from build123d import *

# Parameters (mm, degrees)
BOSS_EXTRU_1_OUTLINE_W   = 46
BOSS_EXTRU_1_OUTLINE_H   = 46
BOSS_EXTRU_1_OUTLINE_W_2 = 5
BOSS_EXTRU_1_OUTLINE_H_2 = 5
BOSS_EXTRU_1_OUTLINE_R   = 5
BOSS_EXTRU_1_DEPTH       = 5
CONG_1_R                 = 3


# Read off the part's stored shape, not the designer's step: Boss.-Extru.1
with BuildPart() as part:
    # Boss.-Extru.1 outline → Boss.-Extru.1 (new body)
    with BuildSketch(Plane.XY):
        with Locations((0, 23)):
            Rectangle(BOSS_EXTRU_1_OUTLINE_W, BOSS_EXTRU_1_OUTLINE_H)
        with Locations((-7.5, 5.5)):
            Rectangle(BOSS_EXTRU_1_OUTLINE_W_2, BOSS_EXTRU_1_OUTLINE_H_2, mode=Mode.SUBTRACT)
        with Locations((-17.5, 15.5)):
            Rectangle(BOSS_EXTRU_1_OUTLINE_W_2, BOSS_EXTRU_1_OUTLINE_H_2, mode=Mode.SUBTRACT)
        with Locations((7.5, 5.5)):
            Rectangle(BOSS_EXTRU_1_OUTLINE_W_2, BOSS_EXTRU_1_OUTLINE_H_2, mode=Mode.SUBTRACT)
        with Locations((17.5, 15.5)):
            Rectangle(BOSS_EXTRU_1_OUTLINE_W_2, BOSS_EXTRU_1_OUTLINE_H_2, mode=Mode.SUBTRACT)
        with Locations((-17.5, 30.5)):
            Rectangle(BOSS_EXTRU_1_OUTLINE_W_2, BOSS_EXTRU_1_OUTLINE_H_2, mode=Mode.SUBTRACT)
        with Locations((-7.5, 40.5)):
            Rectangle(BOSS_EXTRU_1_OUTLINE_W_2, BOSS_EXTRU_1_OUTLINE_H_2, mode=Mode.SUBTRACT)
        with Locations((0, 25)):
            Circle(BOSS_EXTRU_1_OUTLINE_R, mode=Mode.SUBTRACT)
        with Locations((17.5, 30.5)):
            Rectangle(BOSS_EXTRU_1_OUTLINE_W_2, BOSS_EXTRU_1_OUTLINE_H_2, mode=Mode.SUBTRACT)
        with Locations((7.5, 40.5)):
            Rectangle(BOSS_EXTRU_1_OUTLINE_W_2, BOSS_EXTRU_1_OUTLINE_H_2, mode=Mode.SUBTRACT)
    extrude(amount=BOSS_EXTRU_1_DEPTH)

    # Congé1
    cong_1_edges = [part.edges().sort_by_distance(p)[0] for p in [
        (-23, 0, 2.5),
        (-23, 46, 2.5),
        (23, 46, 2.5),
        (23, 0, 2.5),
    ]]
    fillet(cong_1_edges, radius=CONG_1_R)


solid = part.part
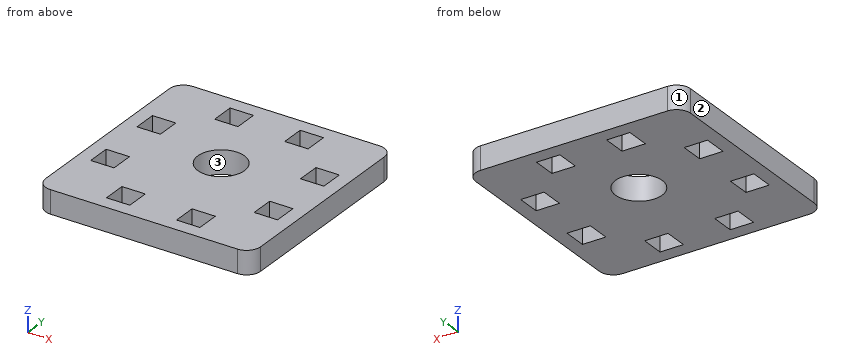
Read the model definition and answer for the solid it produces. Units are mm, in the model's axes. Face numbers are marked on the shaded views. Coordinates: 2 decimals unless noted, no trailing zeros. Write each loop counter-clockwise with the first axis right and the second up, starting at its lowest first coordinate (ties: lowest second). Pieces come first, ordered by that corner, then holes. Notation, with made-up numbers: (-18.5, 54) - (31.5, 54) arc R18 ccw to (31.5, 62) - close; hole circle Ø2 at (-24.5, -26.5). An arc over 180 degrees is marked (long way). One line per question, with ' | ' between items.
Q1. Determine the mould class of the marked faces 1, 2 and 3 for opening direction Y: +Y half, -Y half, draft (parallel to the pull), parting line (faces both ways), or undercut.
Result set:
face 1: +Y half | face 2: draft | face 3: undercut
Q2. Find section D-D, the plane z = 1.2. State how many separate pieces and enclosed holes the cut face has, plus the area to 3 significant figures.
Result set:
separate pieces: 1 | enclosed holes: 9 | area: 1,830 mm^2
Q3. Consider L1, parallel to Y at x = 16.5, z = 3; L2, parallel to Y at x = 8, z = 3.2; L3, parallel to X at y = 40, z = 0.85. Determine where each line is inside the solid, lowest interval first. Write a range as [from, to].
Result set:
L1: [0, 13], [18, 28], [33, 46] | L2: [0, 3], [8, 38], [43, 46] | L3: [-23, -10], [-5, 5], [10, 23]
Q4. Find section A-A, the plane x = 0. Write down the section's boundary in (y, z).
Result set:
outline: (0, 0) - (20, 0) - (20, 5) - (0, 5) - close; (30, 0) - (46, 0) - (46, 5) - (30, 5) - close
Q5. Each of these flat-tipped pins is pushed along its axis until it touches: P1, Ø3, axis at x = -12, y = 27, coming from the -Z side; P2, Ø8, axis at x = 0, y = 25, coming from the +Z side. Where does it stop, or does it pass through?
Result set:
P1: z = 0 | P2: through
Q6. Find section C-C, the plane x = 9. Write down the section's boundary in (y, z), plus the area to 3 significant figures.
Result set:
outline: (0, 0) - (3, 0) - (3, 5) - (0, 5) - close; (8, 0) - (38, 0) - (38, 5) - (8, 5) - close; (43, 0) - (46, 0) - (46, 5) - (43, 5) - close | area: 180 mm^2
Q7. Find section B-B, the plane y = 25. Write down the section's boundary in (x, z).
Result set:
outline: (-23, 0) - (-5, 0) - (-5, 5) - (-23, 5) - close; (5, 0) - (23, 0) - (23, 5) - (5, 5) - close
